```python
from build123d import *

# Parameters (mm, degrees)
F0_W     = 20
F0_H     = 15
F1_DEPTH = 2
F2_W     = 8
F2_H     = 15
F3_DEPTH = 4
F4_R     = 1.25
F5_DEPTH = 15.001
F6_R     = 1
F7_DEPTH = 25
F8_R     = 3


with BuildPart() as f1:
    # F0 (on Top) → F1 (new body)
    with BuildSketch(Plane.XY):
        Rectangle(F0_W, F0_H)
    extrude(amount=F1_DEPTH)

    # F2 (on face) → F3 (join)
    with BuildSketch(Plane.XY.offset(2)):
        Rectangle(F2_W, F2_H)
    extrude(amount=F3_DEPTH)

    # F4 (on face) → F5 (cut, through all)
    with BuildSketch(Plane.XZ.offset(7.5)):
        with Locations((0, 2.75)):
            Circle(F4_R)
    extrude(amount=-F5_DEPTH, mode=Mode.SUBTRACT)

    # F6 (on face) → F7 (cut)
    with BuildSketch(Plane(origin=(0, 0, 0), x_dir=(1, 0, 0), z_dir=(0, 0, -1))):
        with Locations((-7, 4.5)):
            Circle(F6_R)
        with Locations((7, 4.5)):
            Circle(F6_R)
        with Locations((7, -4.5)):
            Circle(F6_R)
        with Locations((-7, -4.5)):
            Circle(F6_R)
    extrude(amount=-F7_DEPTH, mode=Mode.SUBTRACT)

    # F8
    f8_edges = [f1.edges().sort_by_distance(p)[0] for p in [
        (4, 0, 6),
        (-4, 0, 6),
        (10, -7.5, 1),
        (10, 7.5, 1),
        (-10, -7.5, 1),
        (-10, 7.5, 1),
    ]]
    fillet(f8_edges, radius=F8_R)


solid = f1.part
```
Model file for the job. Use its own axes, mm. A direction names the side the tool comes from. Give positions to 0.01 mm unless a question says otherwise; leave off trailing zeros. Loops run counter-clockwise (first coordinate to the right, second up) from the corner with the lowest first, then second, coordinate; pieces in that order, holes last. Notation, with made-up numbers: M -8.5,-28.75 L 26.5,-28.75 A14 ccw 26.5,-17.75 Z; hole C -39.75,67.25 d9. An arc over 180 degrees is marked long. Use one line per item in the form item = value.
Item 1: Two-plate mould, pull along Y, no slides. Class faces 4 (the cylindrical face through (-7.13, -5.49, 0.99)), 5 (the cylindrical face through (9.1, 6.64, 1.01)), 6 (the flat face through (10, 0, 1)): released by +Y, released by -Y, zero draft, split by the parting line, or undercut.
Filled in:
face_4 = undercut
face_5 = released by +Y
face_6 = zero draft
Item 2: Slice it at D-D on y = 3. List the corners of the cut face in (x, z), and give its area (3 significant figures).
Filled in:
outline = M -10,0 L 10,0 L 10,2 L 4,2 L 4,3 A3 ccw 1,6 L -1,6 A3 ccw -4,3 L -4,2 L -10,2 Z; hole C 0,2.75 d2.5
area = 63.2 mm^2
Item 3: Drill centre lines: L1, parallel to X at y = 4.5, z = 0.55; L2, parallel to Y at x = 7, z = 1.3; L3, parallel to X at y = -5.25, z = 0.6. Where is each one in solid material? Low to high.
Filled in:
L1 = -10 to -8, -6 to 6, 8 to 10
L2 = -7.5 to -5.5, -3.5 to 3.5, 5.5 to 7.5
L3 = -9.9 to -7.66, -6.34 to 6.34, 7.66 to 9.9
Item 4: Slice it at A-A on z = 2.75. List the corners of the cut face in (x, y).
Filled in:
outline = M -4,-7.5 L -1.25,-7.5 L -1.25,7.5 L -4,7.5 Z; M 1.25,-7.5 L 4,-7.5 L 4,7.5 L 1.25,7.5 Z
Item 5: Slice it at B-B on y = -4. List the corners of the cut face in (x, z).
Filled in:
outline = M -10,0 L -7.87,0 L -7.87,2 L -10,2 Z; M -6.13,0 L 6.13,0 L 6.13,2 L 4,2 L 4,3 A3 ccw 1,6 L -1,6 A3 ccw -4,3 L -4,2 L -6.13,2 Z; M 7.87,0 L 10,0 L 10,2 L 7.87,2 Z; hole C 0,2.75 d2.5
Item 6: Slice it at C-C on x = 0. List the corners of the cut face in (y, z).
Filled in:
outline = M -7.5,0 L 7.5,0 L 7.5,1.5 L -7.5,1.5 Z; M -7.5,4 L 7.5,4 L 7.5,6 L -7.5,6 Z
Item 7: Flat gauge pins, fed straight in: pin 1 Ø1 at (x, y) = (-7.5, -5) entering from +Z; pin 2 Ø0.5 at (y, z) = (0.5, 2.5) entering from +X; pin 3 Ø0.5 at (y, z) = (3.5, 2.5) entering from -X. Where does each tip first touch, or does it go through?
Filled in:
pin_1 = 2
pin_2 = 4
pin_3 = -4
Item 8: Which spindle directions (+Z, -Z, +X, -X, +Y, -Y) get a long thin tool onto all of the face, cutting with end or side? Do faces 1 (the flat face through (0, 0, 0)), 2 (the flat face through (-7, 0, 2)), 3 (the flat face through (4, -0.1, 2.5)). Say none if no direction does.
Filled in:
face_1 = -Z, +X, -X, +Y, -Y
face_2 = +Z, -X, +Y, -Y
face_3 = +Z, +X, +Y, -Y
